```python
from build123d import *

# Parameters (mm, degrees)
SKETCH1_R           = 1.7
BOSS_EXTRUDE1_DEPTH = 6.985
FILLET1_R           = 6.35


with BuildPart() as part:
    # Sketch1 → Boss-Extrude1 (new body)
    with BuildSketch(Plane(origin=(0, 0, 0), x_dir=(1, 0, 0), z_dir=(0, 1, 0))):
        Polygon((-72.39, 6.35), (-72.39, -6.35), (-6.35, -6.35), (6.35, -6.35), (72.39, -6.35), (72.39, 6.35), (6.35, 6.35), (-6.35, 6.35), align=None)
        with Locations(Location((-66.04, 0, 0), (0, 0, 270))):
            Circle(SKETCH1_R, mode=Mode.SUBTRACT)
        with Locations(Location((66.04, 0, 0), (0, 0, 270))):
            Circle(SKETCH1_R, mode=Mode.SUBTRACT)
    extrude(amount=BOSS_EXTRUDE1_DEPTH)

    # Fillet1
    fillet1_edges = [part.edges().sort_by_distance(p)[0] for p in [
        (72.39, 3.4925, -6.35),
        (-72.39, 3.4925, -6.35),
        (-72.39, 3.4925, 6.35),
        (72.39, 3.4925, 6.35),
    ]]
    fillet(fillet1_edges, radius=FILLET1_R - 0.0001)  # a hair under: the kernel refuses the full size


solid = part.part
```
For this review, take the finished solid that the model builds, in its own axes (mm). Coordinates: 2 decimals unless noted, no trailing zeros. Loops run counter-clockwise (first coordinate to the right, second up) from the corner with the lowest first, then second, coordinate; pieces in that order, holes last.
1. Add section A-A, the plane y = 2. Count the separate pieces of the cut face and the enclosed holes in it, then the cut area to 3 significant figures.
2. Insertion check: P1, Ø4, axis at x = 66.04, z = 0, coming from the -Y side; P2, Ø1, axis at y = 5, z = 1, coming from the +X side; P3, Ø3, axis at y = 2, z = -4.5, coming from the +X side. Each pin has a flat end and moves straight along its axis. Give the tip position at first contact, or say it passes through.
3. For line 1 (X direction, y = 5.5, z = 0); line 2 (Z direction, x = 66.04, y = 1.75); line 3 (X direction, y = 4, z = 0.5), list the stretches that pass through material, from the lowest coordinate up.
4. Add section C-C, the plane z = 4.25. Give the boundary of the cut face in (x, y) (3 decimals), then the cut area to 3 significant figures.
5. Add section B-B, the plane z = -5. Give the boundary of the cut face in (x, y) (3 decimals), then the cut area to 3 significant figures.
6. Mouldability with a two-part tool opening along X and no side actions: class faces 1 (the cylindrical face through (70.48, 3.54, 4.54)), 2 (the flat face through (-1, 0, 0)), 3 (the cylindrical face through (64.38, 3.44, -0.37)) as +X half, -X half, draft (parallel to the pull), parting line (faces both ways), or undercut.
Result:
1. separate pieces: 1
1. enclosed holes: 2
1. area: 1,790 mm2
2. P1: stops at y = 0
2. P2: stops at x = 72.37
2. P3: stops at x = 71.64
3. line 1: x = -72.39 to -67.74, -64.34 to 64.34, 67.74 to 72.39
3. line 2: z = -6.35 to -1.7, 1.7 to 6.35
3. line 3: x = -72.37 to -67.66, -64.42 to 64.42, 67.66 to 72.37
4. outline: (-70.758, 0) - (70.758, 0) - (70.758, 6.985) - (-70.758, 6.985) - close
4. area: 988 mm2
5. outline: (-69.954, 0) - (69.954, 0) - (69.954, 6.985) - (-69.954, 6.985) - close
5. area: 977 mm2
6. face 1: +X half
6. face 2: draft
6. face 3: undercut
